```python
from build123d import *

# Parameters (mm, degrees)
BOSS_EXTRUDE1_DEPTH = 3
SKETCH3_R           = 1.75
CUT_EXTRUDE1_DEPTH  = 3
SKETCH5_R           = 3
CUT_EXTRUDE2_DEPTH  = 2


with BuildPart() as part:
    # Sketch2 → Boss-Extrude1 (new body)
    with BuildSketch(Plane.XY):
        with BuildLine():
            Line((-5.255475961, 15.75), (-0.965925826, -0.258819045))
            ThreePointArc((-0.965925826, -0.258819045), (0, -1), (0.965925826, -0.258819045))
            Line((0.965925826, -0.258819045), (5.255475961, 15.75))
            Line((5.255475961, 15.75), (10, 15.75))
            Line((10, 15.75), (10, 25.75))
            Line((10, 25.75), (-10, 25.75))
            Line((-10, 25.75), (-10, 15.75))
            Line((-10, 15.75), (-5.255475961, 15.75))
        make_face()
    extrude(amount=BOSS_EXTRUDE1_DEPTH)

    # Sketch3 → Cut-Extrude1 (cut)
    with BuildSketch(Plane.XY.offset(3)):
        with Locations((-5, 20.75)):
            Circle(SKETCH3_R)
        with Locations((5, 20.75)):
            Circle(SKETCH3_R)
    extrude(amount=-CUT_EXTRUDE1_DEPTH, mode=Mode.SUBTRACT)

    # Sketch5 → Cut-Extrude2 (cut)
    with BuildSketch(Plane.XY.offset(3)):
        with Locations((-5, 20.75)):
            Circle(SKETCH5_R)
        with Locations(Location((5, 20.75, 0), (0, 0, 180))):
            Circle(SKETCH5_R)
    extrude(amount=-CUT_EXTRUDE2_DEPTH, mode=Mode.SUBTRACT)


solid = part.part
```
Could you check a few things on this model? Use its own coordinates, in mm. A direction names the side the tool comes from. Round coordinates to 2 decimals unless told otherwise and drop trailing zeros. Loops run counter-clockwise (first coordinate to the right, second up) from the corner with the lowest first, then second, coordinate; pieces in that order, holes last. Notation, with made-up numbers: M 53.5,3.5 L 68.5,3.5 A10 ccw 68.5,19.5 Z; hole C -3.75,-21.5 d9. An arc over 180 degrees is marked long. Put each result on its own line as item: value.
Q1. Thinking about a two-plate mould opening in Y: for faces 6 (the face through (4.772, 22.485, 0.507)), 7 (the face through (-10, 21, 1)), 8 (the face through (-3.14, 7.86, 1.48)), 9 (the face through (5, 23, 1)), which applies, released by +Y, released by -Y, zero draft, split by the parting line, or undercut?
Check result:
face 6: undercut
face 7: zero draft
face 8: released by -Y
face 9: undercut
Q2. Imagine slicing it at D-D (y = 1). Write out the boundary of the cut face in (x, z).
Check result:
outline: M -1.3,0 L 1.3,0 L 1.3,3 L -1.3,3 Z
Q3. I need wall thicknesses on probe 1 along X at (y, z) = (18.75, 1.4); probe 2 along X at (y, z) = (22.25, 2.2); probe 3 along Y at (x, z) = (-7.25, 0.85). Which ranges of each line are inside material? Lowest first, please.
Check result:
probe 1: -10 to -7.24, -2.76 to 2.76, 7.24 to 10
probe 2: -10 to -7.6, -2.4 to 2.4, 7.6 to 10
probe 3: 15.75 to 25.75
Q4. Imagine slicing it at C-C (x = -4.75). Write out the boundary of the cut face in (y, z).
Check result:
outline: M 13.86,0 L 19.02,0 L 19.02,1 L 17.76,1 L 17.76,3 L 13.86,3 Z; M 22.48,0 L 25.75,0 L 25.75,3 L 23.74,3 L 23.74,1 L 22.48,1 Z
Q5. Imagine slicing it at B-B (z = 2.2). Write out the boundary of the cut face in (x, y).
Check result:
outline: M -10,15.75 L -5.26,15.75 L -0.97,-0.26 A1 ccw 0.97,-0.26 L 5.26,15.75 L 10,15.75 L 10,25.75 L -10,25.75 Z; hole C -5,20.75 d6; hole C 5,20.75 d6
Q6. On a 3-axis mill with a long thin cutter (end or side, diameter ignored), from which of +Z, -Z, +X, -X, +Y, -Y can I reach the whole of each face in a straight line? I mean faces 1 (the face through (0, -1, 1)), 2 (the face through (-4, 19, 1)), 3 (the face through (8, 15.75, 1)), 4 (the face through (-8, 15.75, 1)), 5 (the face through (-5.228, 22.485, 0.507)). Say none if no direction works.
Check result:
face 1: +Z, -Z, -Y
face 2: +Z
face 3: +Z, -Z, +X, -Y
face 4: +Z, -Z, -X, -Y
face 5: +Z, -Z
Q7. Imagine slicing it at A-A (y = 20.75). Write out the boundary of the cut face in (x, z).
Check result:
outline: M -10,0 L -6.75,0 L -6.75,1 L -8,1 L -8,3 L -10,3 Z; M -3.25,0 L 3.25,0 L 3.25,1 L 2,1 L 2,3 L -2,3 L -2,1 L -3.25,1 Z; M 6.75,0 L 10,0 L 10,3 L 8,3 L 8,1 L 6.75,1 Z
Q8. For pin 1 (1.5 mm diameter, centred on x = 8.5, z = 1.5, fed in from -Y); pin 2 (4.5 mm diameter, centred on x = 5, y = 20.75, fed in from +Z), each with a flat end and sliding along its axis, tell me the tip position at first contact or that it passes through.
Check result:
pin 1: y = 15.75
pin 2: z = 1
